Check sheet for the modelled part. Datum: model origin and axes. Units: mm. Round coordinates to 2 decimals unless told otherwise and drop trailing zeros. Order: outer loops, then holes, each group sorted by start corner. A loop starts at its lowest first (then second) coordinate and runs counter-clockwise, first axis right, second up. Notation, with made-up numbers: (50.25, 15) -> (82.25, 15) arc R23 ccw to (82.25, 40) -> close; hole circle Ø4 at (42.25, -6). An arc over 180 degrees is marked (long way). Use CSV: the item, a comma, the result in double quotes.
```python
from build123d import *

# Parameters (mm, degrees)
SKETCH1_R           = 2.1828125
BOSS_EXTRUDE1_DEPTH = 0.79375
FILLET1_R           = 6.35
FILLET2_R           = 3.175
FILLET3_R           = 1.5875


with BuildPart() as part:
    # Sketch1 → Boss-Extrude1 (new body, symmetric)
    with BuildSketch(Plane.XY):
        Polygon((0, 0), (-152.4, 0), (-12.7, 76.2), align=None)
        with Locations((-7.495923678, 6.35)):
            Circle(SKETCH1_R, mode=Mode.SUBTRACT)
        with Locations((-121.795923678, 6.35)):
            Circle(SKETCH1_R, mode=Mode.SUBTRACT)
    extrude(amount=BOSS_EXTRUDE1_DEPTH, both=True)

    # Fillet1
    fillet1_edges = [part.edges().sort_by_distance(p)[0] for p in [
        (0, 0, 0),
    ]]
    fillet(fillet1_edges, radius=FILLET1_R)

    # Fillet2
    fillet2_edges = [part.edges().sort_by_distance(p)[0] for p in [
        (-12.7, 76.2, 0),
    ]]
    fillet(fillet2_edges, radius=FILLET2_R)

    # Fillet3
    fillet3_edges = [part.edges().sort_by_distance(p)[0] for p in [
        (-152.4, 0, 0),
    ]]
    fillet(fillet3_edges, radius=FILLET3_R)


solid = part.part
```
Q1. Sectioned sample at B-B, the plane y = 13.5. Enter the section's corners in (x, z).
Result sheet:
outline,"(-127.65, -0.79) -> (-2.25, -0.79) -> (-2.25, 0.79) -> (-127.65, 0.79) -> close"
Q2. Sectioned sample at A-A, the plane z = -0.35. State how many separate pieces and enclosed holes the cut face has, then the cut area to 3 significant figures.
Result sheet:
separate pieces,"1"
enclosed holes,"2"
area,"5,750 mm^2"
Q3. Sectioned sample at C-C, the plane x = -128.5. Enter the section's corners in (y, z), then the cut area to 3 significant figures.
Result sheet:
outline,"(0, -0.79) -> (13.04, -0.79) -> (13.04, 0.79) -> (0, 0.79) -> close"
area,"20.7 mm^2"
Q4. Go/stop test with a flat-tipped pin: pin 1 (2.5 mm diameter, centred on x = -7.5, y = 6.35, fed in from +Z). Record where the tip stops, or that it passes through.
Result sheet:
pin 1,"passes through"
Q5. Scan lines: L1, parallel to Y at x = -91, z = -0.65; L2, parallel to Y at x = -49.5, z = 0.55; L3, parallel to X at y = 56, z = -0.2. Record each from-to range of solid material in increasing order.
Result sheet:
L1,"y = 0 to 33.49"
L2,"y = 0 to 56.13"
L3,"x = -49.73 to -9.33"
Q6. Mould release check, pull along X, two halves, no side actions. Record for faces 1 (the face through (-57, 21, -0.794)), 2 (the face through (-123.977, 6.446, -0.011)), 3 (the face through (-13.75, 74.15, 0.01)), 4 (the face through (-2.7, 2.19, 0.01)): pulls with the +X half, pulls with the -X half, needs draft (parallel to the pull), parting line crosses it, or undercut.
Result sheet:
face 1,"needs draft"
face 2,"undercut"
face 3,"parting line crosses it"
face 4,"pulls with the +X half"
